from build123d import *

# Parameters (mm, degrees)
SKETCH1_W                      = 316
SKETCH1_H                      = 230
BASE_FLANGE1_DEPTH             = 10
EDGE_FLANGE1_STRIP_W           = 70
EDGE_FLANGE1_STRIP_H           = 10
EDGE_FLANGE1_STRIP_CUT_DEPTH   = 230
EDGE_FLANGE1_STRIP_2_W         = 70
EDGE_FLANGE1_STRIP_2_H         = 10
EDGE_FLANGE1_STRIP_CUT_2_DEPTH = 230
EDGE_FLANGE1_DEPTH             = 230
EDGE_FLANGE1_BEND_DEPTH        = 230
SKETCH12_R                     = 27.5
CUT_EXTRUDE1_DEPTH             = 10
SKETCH14_R                     = 9.5
CUT_EXTRUDE3_DEPTH             = 10
CIRPATTERN1_COUNT              = 4
SKETCH17_R                     = 7
CUT_EXTRUDE4_DEPTH             = 420.023865669


# Sheet-metal steps are written as plain solids
with BuildPart() as part:
    # Sketch1 → Base-Flange1 (new body)
    with BuildSketch(Plane(origin=(0, 0, 0), x_dir=(0, 0, -1), z_dir=(1, 0, 0))):
        Rectangle(SKETCH1_W, SKETCH1_H)
    extrude(amount=-BASE_FLANGE1_DEPTH)

    # Edge-Flange1 strip (across the edge) → Edge-Flange1 strip cut (cut)
    with BuildSketch(Plane(origin=(-10, -115, 158), x_dir=(0, 0, -1), z_dir=(0, 1, 0))):
        with Locations((-10, -5)):
            Rectangle(EDGE_FLANGE1_STRIP_W, EDGE_FLANGE1_STRIP_H)
    extrude(amount=EDGE_FLANGE1_STRIP_CUT_DEPTH, mode=Mode.SUBTRACT)

    # Edge-Flange1 strip 2 (across the edge) → Edge-Flange1 strip cut 2 (cut)
    with BuildSketch(Plane(origin=(-10, 115, -158), x_dir=(0, 0, 1), z_dir=(0, -1, 0))):
        with Locations((-10, -5)):
            Rectangle(EDGE_FLANGE1_STRIP_2_W, EDGE_FLANGE1_STRIP_2_H)
    extrude(amount=EDGE_FLANGE1_STRIP_CUT_2_DEPTH, mode=Mode.SUBTRACT)

    # Edge-Flange1 section (across the edge) → Edge-Flange1 (add)
    with BuildSketch(Plane(origin=(-10, -115, 158), x_dir=(0, 0, -1), z_dir=(0, 1, 0))):
        with BuildLine():
            Line((0, 15), (0, 240))
            Line((0, 240), (10, 240))
            Line((10, 240), (10, 15))
            ThreePointArc((10, 15), (14.393398282, 4.393398282), (25, 0))
            Line((25, 0), (25, -10))
            ThreePointArc((25, -10), (7.32233047, -2.67766953), (0, 15))
        make_face()
    extrude(amount=EDGE_FLANGE1_DEPTH)

    # Edge-Flange1 section 2 (across the edge) → Edge-Flange1 bend (add)
    with BuildSketch(Plane(origin=(-10, 115, -158), x_dir=(0, 0, 1), z_dir=(0, -1, 0))):
        with BuildLine():
            Line((0, 15), (0, 240))
            Line((0, 240), (10, 240))
            Line((10, 240), (10, 15))
            ThreePointArc((10, 15), (14.393398282, 4.393398282), (25, 0))
            Line((25, 0), (25, -10))
            ThreePointArc((25, -10), (7.32233047, -2.67766953), (0, 15))
        make_face()
    extrude(amount=EDGE_FLANGE1_BEND_DEPTH)

    # Sketch12 → Cut-Extrude1 (cut)
    with BuildSketch(Plane(origin=(0, 0, 0), x_dir=(0, 0, -1), z_dir=(1, 0, 0))):
        Circle(SKETCH12_R)
    extrude(amount=-CUT_EXTRUDE1_DEPTH, mode=Mode.SUBTRACT)

    # Sketch14 → Cut-Extrude3 (cut)
    with BuildSketch(Plane(origin=(0, 0, 0), x_dir=(0, 0, -1), z_dir=(1, 0, 0))):
        with Locations((-50, 50)):
            Circle(SKETCH14_R)
    cut_extrude3 = extrude(amount=-CUT_EXTRUDE3_DEPTH, mode=Mode.SUBTRACT)

    # CirPattern1: Cut-Extrude3 ×4 about axis
    cirpattern1_axis = Axis((0, 0, 0), (1, 0, 0))
    for i in range(1, CIRPATTERN1_COUNT):
        add(cut_extrude3.rotate(cirpattern1_axis, i * 360 / CIRPATTERN1_COUNT), mode=Mode.SUBTRACT)

    # Sketch17 → Cut-Extrude4 (cut, through all)
    with BuildSketch(Plane.XY.offset(158)):
        with Locations((-229, 60)):
            Circle(SKETCH17_R)
        with Locations((-229, -60)):
            Circle(SKETCH17_R)
    extrude(amount=-CUT_EXTRUDE4_DEPTH, mode=Mode.SUBTRACT)


solid = part.part
Design review of the part built by this model. Coordinates are the model's own, in mm. A direction names the side the tool comes from. Coordinates: 2 decimals unless noted, no trailing zeros. Loops run counter-clockwise (first coordinate to the right, second up) from the corner with the lowest first, then second, coordinate; pieces in that order, holes last.
Item 1: Draft analysis for pull direction Y (two halves, no side actions). For faces 3 (the cylindrical face through (-14.51, -1.61, 143.72)), 4 (the flat face through (-5, -115, 1)), 5 (the cylindrical face through (-4.93, 58.01, 44.89)), state which applies: pulls with the +Y half, pulls with the -Y half, needs draft (parallel to the pull), parting line crosses it, or undercut.
Completed:
face 3: needs draft
face 4: pulls with the -Y half
face 5: undercut
Item 2: Add section B-B (z = 50). Write out the cut boundary in (x, y).
Completed:
outline: (-10, -115) - (0, -115) - (0, -59.5) - (-10, -59.5) - close; (-10, -40.5) - (0, -40.5) - (0, 40.5) - (-10, 40.5) - close; (-10, 59.5) - (0, 59.5) - (0, 115) - (-10, 115) - close
Item 3: For faces 1 (the flat face through (-10, 2, 31)), 2 (the cylindrical face through (-222.323, 62.103, -152.93)), list the 3-axis set-ups (+Z, -Z, +X, -X, +Y, -Y) from which the entire face can be reached by the end or side of a thin tool; tool diameter is ignored.
Completed:
face 1: -X, +Y, -Y
face 2: +Z, -Z
Item 4: Clearance check with flat-ended pins moving along their axes: pin 1 (6 mm diameter, centred on y = 37, z = -110, fed in from +X); pin 2 (24.5 mm diameter, centred on y = -50, z = -50, fed in from -X). State where each tip first meets the part, or that it passes through.
Completed:
pin 1: stops at x = 0
pin 2: stops at x = -10
Item 5: Add section D-D (z = 8). Write out the cut boundary in (x, y).
Completed:
outline: (-10, -115) - (0, -115) - (0, -26.31) - (-10, -26.31) - close; (-10, 26.31) - (0, 26.31) - (0, 115) - (-10, 115) - close
Item 6: Add section A-A (x = -229). Write out the cut boundary in (y, z), and give its area (3 significant figures).
Completed:
outline: (-115, -158) - (-67, -158) - (-67, -148) - (-115, -148) - close; (-115, 148) - (-67, 148) - (-67, 158) - (-115, 158) - close; (-53, -158) - (53, -158) - (53, -148) - (-53, -148) - close; (-53, 148) - (53, 148) - (53, 158) - (-53, 158) - close; (67, -158) - (115, -158) - (115, -148) - (67, -148) - close; (67, 148) - (115, 148) - (115, 158) - (67, 158) - close
area: 4,040 mm2
Item 7: Add section C-C (x = -140). Write out the cut boundary in (y, z).
Completed:
outline: (-115, -158) - (115, -158) - (115, -148) - (-115, -148) - close; (-115, 148) - (115, 148) - (115, 158) - (-115, 158) - close
Item 8: Wall thickness on L1, parallel to Y at x = -229, z = -153; L2, parallel to Y at x = -3.75, z = -50; L3, parallel to Z at x = -169.5, y = -60: over which ranges is each line inside the solid? List them lowest first.
Completed:
L1: y = -115 to -67, -53 to 53, 67 to 115
L2: y = -115 to -59.5, -40.5 to 40.5, 59.5 to 115
L3: z = -158 to -148, 148 to 158
